```python
from build123d import *

# Parameters (mm, degrees)
F0_W     = 3.95
F0_H     = 3
F1_DEPTH = 3.9
F0_W_2   = 6.5
F0_H_2   = 5
F2_DEPTH = 100
F3_W     = 4
F3_H     = 3.077
F3_W_2   = 3.25
F3_H_2   = 5
F4_DEPTH = 4
F5_R     = 2.7


with BuildPart() as f1:
    # F0 (on Top) → F1 (new body)
    with BuildSketch(Plane.XY):
        with Locations((-28.5066142678, -30.1459487528)):
            Rectangle(F0_W, F0_H)
    extrude(amount=-F1_DEPTH)

    # F0 (on Top) → F2 (join)
    with BuildSketch(Plane.XY):
        with Locations((-28.5066142678, -30.1459487528)):
            Rectangle(F0_W_2, F0_H_2)
        with Locations((-28.5066142678, -30.1459487528)):
            Rectangle(F0_W, F0_H, mode=Mode.SUBTRACT)
        with Locations((-28.5066142678, -30.1459487528)):
            Rectangle(F0_W, F0_H)
    extrude(amount=F2_DEPTH)

    # F3 (on face) → F4 (join)
    with BuildSketch(Plane.XY.offset(100)):
        Polygon((-64.0066142678, -2.6459487528), (-31.7566142678, -32.6459487528), (-31.7566142678, -27.6459487528), (-28.5066142678, -27.6459487528), (-28.5066142678, -7.6844487528), (-30.5066142678, -7.6844487528), (-30.5066142678, -4.6074487528), (-28.5066142678, -4.6074487528), (-28.5066142678, -2.6459487528), align=None)
        with Locations((-54.7566142678, -6.1459487528)):
            Rectangle(F3_W, F3_H, mode=Mode.SUBTRACT)
        Polygon((6.9933857322, -2.6459487528), (-28.5066142678, -2.6459487528), (-28.5066142678, -4.6074487528), (-26.5066142678, -4.6074487528), (-26.5066142678, -7.6844487528), (-28.5066142678, -7.6844487528), (-28.5066142678, -27.6459487528), (-25.2566142678, -27.6459487528), (-25.2566142678, -32.6459487528), align=None)
        with Locations((-2.2566142678, -6.1459487528)):
            Rectangle(F3_W, F3_H, mode=Mode.SUBTRACT)
        with Locations((-26.8816142678, -30.1459487528)):
            Rectangle(F3_W_2, F3_H_2)
        with Locations((-30.1316142678, -30.1459487528)):
            Rectangle(F3_W_2, F3_H_2)
    extrude(amount=F4_DEPTH)

    # F5
    f5_edges = [f1.edges().sort_by_distance(p)[0] for p in [
        (-64.006614, -2.645949, 102),
        (6.993386, -2.645949, 102),
    ]]
    fillet(f5_edges, radius=F5_R)


solid = f1.part
```
The model under review builds one solid part; all positions refer to its coordinate system, in mm. A direction names the side the tool comes from. Round coordinates to 2 decimals unless told otherwise and drop trailing zeros. Order: outer loops, then holes, each group sorted by start corner. A loop starts at its lowest first (then second) coordinate and runs counter-clockwise, first axis right, second up.
Item 1: Add section D-D, the plane x = -39. State the section outline as (y, z) points.
Working result:
outline: (-25.91, 100) - (-2.65, 100) - (-2.65, 104) - (-25.91, 104) - close
Item 2: Add section C-C, the plane z = 52.5. State the section outline as (x, y) points.
Working result:
outline: (-31.76, -32.65) - (-25.26, -32.65) - (-25.26, -27.65) - (-31.76, -27.65) - close
Item 3: Draft analysis for pull direction Y (two halves, no side actions). For faces 4 (the flat face through (-31.757, -30, 49)), 5 (the flat face through (-2, -4.607, 102)), 6 (the flat face through (-11.836, -20.162, 101.972)), state which applies: released by +Y, released by -Y, zero draft, split by the parting line, or undercut.
Working result:
face 4: zero draft
face 5: undercut
face 6: released by -Y
Item 4: For pin 1 (8 mm diameter, centred on y = -28, z = 17, fed in from -X); pin 2 (4 mm diameter, centred on x = -31.5, y = -21.5, fed in from -Z); pin 3 (2 mm diameter, centred on x = -28, z = -2.5, fed in from +Y); pin 4 (10 mm diameter, centred on x = -40.5, z = 55, fed in from +Y), all flat-tipped, find the tip position at first contact; note any pin that passes through.
Working result:
pin 1: stops at x = -31.76
pin 2: stops at z = 100
pin 3: stops at y = -28.65
pin 4: passes through
Item 5: Add section B-B, the plane y = -30. State the section outline as (x, z) points.
Working result:
outline: (-34.6, 100) - (-31.76, 100) - (-31.76, 0) - (-30.48, 0) - (-30.48, -3.9) - (-26.53, -3.9) - (-26.53, 0) - (-25.26, 0) - (-25.26, 100) - (-22.41, 100) - (-22.41, 104) - (-34.6, 104) - close
Item 6: To check wall thickness, follow probe 1 along Z at (x, y) = (-32.5, -6); probe 2 along Y at (x, z) = (-25.5, 95); probe 3 along X at (y, z) = (-29, 43). State the ranges of each line that lie inside material, in increasing order.
Working result:
probe 1: z = 100 to 104
probe 2: y = -32.65 to -27.65
probe 3: x = -31.76 to -25.26
Item 7: Add section A-A, the plane x = -3. State the section outline as (y, z) points.
Working result:
outline: (-11.94, 100) - (-7.68, 100) - (-7.68, 104) - (-11.94, 104) - close; (-4.61, 100) - (-2.65, 100) - (-2.65, 104) - (-4.61, 104) - close
Item 8: Machinability: for faces 1 (the flat face through (-4.257, -6, 102)), 2 (the flat face through (-30.482, -30, -2)), 3 (the flat face through (-29, -31.646, -2)), which of the approach directions +Z, -Z, +X, -X, +Y, -Y give a long, thin tool a straight path to every point of the face, cutting with its end or side? Answer none if there is none.
Working result:
face 1: +Z, -Z
face 2: -Z, -X, +Y, -Y
face 3: -Z, +X, -X, -Y
